Source: three-view drawing plus pictorial views. Frame: mm from the lowest corner of the part. A direction names the side the tool comes from. Give positions to 0.01 mm unless a question says otherwise; leave off trailing zeros. Loops run counter-clockwise (first coordinate to the right, second up) from the corner with the lowest first, then second, coordinate; pieces in that order, holes last.
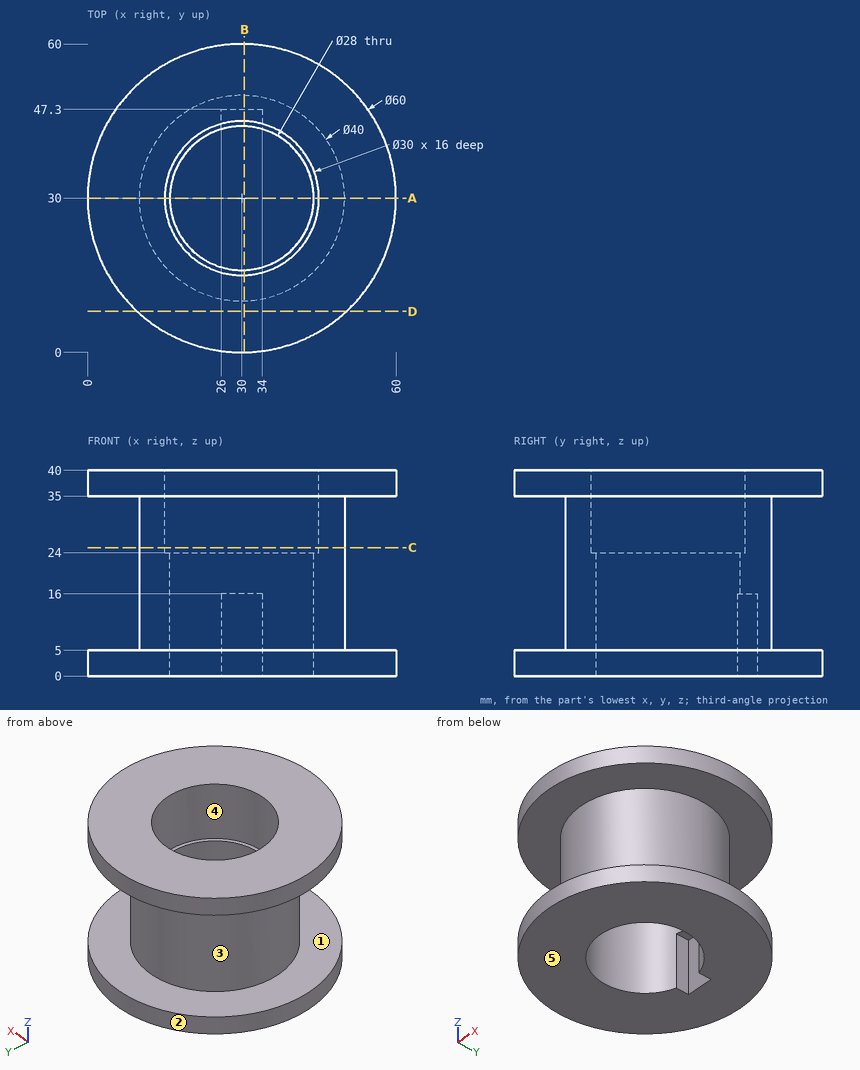
Q1. Section query D-D, the plane y = 8. Return loops of the section in (x, z).
Q2. Mould query, pull axis Z, two halves, no side actions, for the marked faces 3, 4 and 5. Classes: +Z half, -Z half, draft (parallel to the pull), parting line (faces both ways), or undercut.
Q3. Section query B-B, the plane x = 30.5. Return loops of the section in (y, z).
Q4. Pin query (flat end, axial travel): pin 1 Ø1.9 at (y, z) = (45, 5.5) entering from -X; pin 2 Ø12 at (x, z) = (25, 28.5) entering from +Y; pin 3 Ø1.5 at (y, z) = (35.5, 27.5) entering from +X; pin 4 Ø25 at (x, y) = (30, 30) entering from -Z. Return the tip coordinate at first contact, or that it passes through.
Q5. Reachability of the marked faces 1 and 2 from +Z, -Z, +X, -X, +Y, -Y: full face, straight path, thin tool, end or side. Return the list, or none.
Q6. Material intervals for probe 1 along Z at (x, y) = (10, 47.5); probe 2 along Y at (x, z) = (30, 6.25); probe 3 along Y at (x, z) = (30, 19.25), sorted ascending.
Q7. Section query A-A, the plane y = 30. Return loops of the section in (x, z).
Q8. Section query C-C, the plane z = 25. Return loops of the section in (x, y), and give its area (3 significant figures).
Resolved:
1. outline: (9.6, 0) - (50.4, 0) - (50.4, 5) - (9.6, 5) - close; (9.6, 35) - (50.4, 35) - (50.4, 40) - (9.6, 40) - close
2. face 3: undercut
2. face 4: draft
2. face 5: -Z half
3. outline: (0, 0) - (16.01, 0) - (16.01, 24) - (15.01, 24) - (15.01, 40) - (0, 40) - (0, 35) - (10.01, 35) - (10.01, 5) - (0, 5) - close; (43.99, 16) - (47.3, 16) - (47.3, 0) - (60, 0) - (60, 5) - (49.99, 5) - (49.99, 35) - (60, 35) - (60, 40) - (44.99, 40) - (44.99, 24) - (43.99, 24) - close
4. pin 1: stops at x = 3.57
4. pin 2: stops at y = 50
4. pin 3: stops at x = 49.43
4. pin 4: passes through
5. face 1: none
5. face 2: +Z, -Z
6. probe 1: z = 0 to 5, 35 to 40
6. probe 2: y = 10 to 16, 47.3 to 50
6. probe 3: y = 10 to 16, 44 to 50
7. outline: (0, 0) - (16, 0) - (16, 24) - (15, 24) - (15, 40) - (0, 40) - (0, 35) - (10, 35) - (10, 5) - (0, 5) - close; (44, 0) - (60, 0) - (60, 5) - (50, 5) - (50, 35) - (60, 35) - (60, 40) - (45, 40) - (45, 24) - (44, 24) - close
8. outline: circle Ø40 at (30, 30); hole circle Ø30 at (30, 30)
8. area: 550 mm2
